For this review, use the dimensioned drawing (mm, ordinates from the lowest corner) and the shaded views. A direction names the side the tool comes from. Round coordinates to 2 decimals unless told otherwise and drop trailing zeros. Write each loop counter-clockwise with the first axis right and the second up, starting at its lowest first coordinate (ties: lowest second). Pieces come first, ordered by that corner, then holes. Notation, with made-up numbers: M 41,-27 L 84,-27 A29 cw 84,-4 Z; hole C 17,34.5 d5. An arc over 180 degrees is marked long. Use one line per item in the form item = value. Start each with the question number.
Item 1: Add section C-C (x = 63.5). State the section outline as (y, z) points (3 decimals), and give its area (3 significant figures).
Item 2: Add section B-B (x = 47). State the section outline as (y, z) points.
Item 3: For line 1 (Z direction, x = 63.5, y = 1.75) (3 decimals); line 2 (Z direction, x = 63.5, y = 22.5); line 3 (Y direction, x = 27, z = 11.5), list the stretches that pass through material, from the lowest coordinate up. Write a range as [from, to].
Item 4: Add section A-A (z = 60.96). State the section outline as (x, y) points (3 decimals).
Item 5: For P1, Ø8, axis at x = 61, z = 35.5, coming from the +Y side; P2, Ø7, axis at y = 3.5, z = 52.5, coming from the -X side; P3, Ø4, axis at x = 31.5, y = 20, coming from the +Z side, all flat-tipped, find the tip position at first contact; note any pin that passes through.
Item 6: Add section D-D (z = 8). State the section outline as (x, y) points.
Item 7: Draft analysis for pull direction Z (two halves, no side actions). For the marked faces 1, 2 and 3, state which applies: released by +Z, released by -Z, zero draft, split by the parting line, or undercut.
Item 8: For the marked faces 4, 5, 6 and 7, list the 3-axis set-ups (+Z, -Z, +X, -X, +Y, -Y) from which the entire face can be reached by the end or side of a thin tool; tool diameter is ignored.
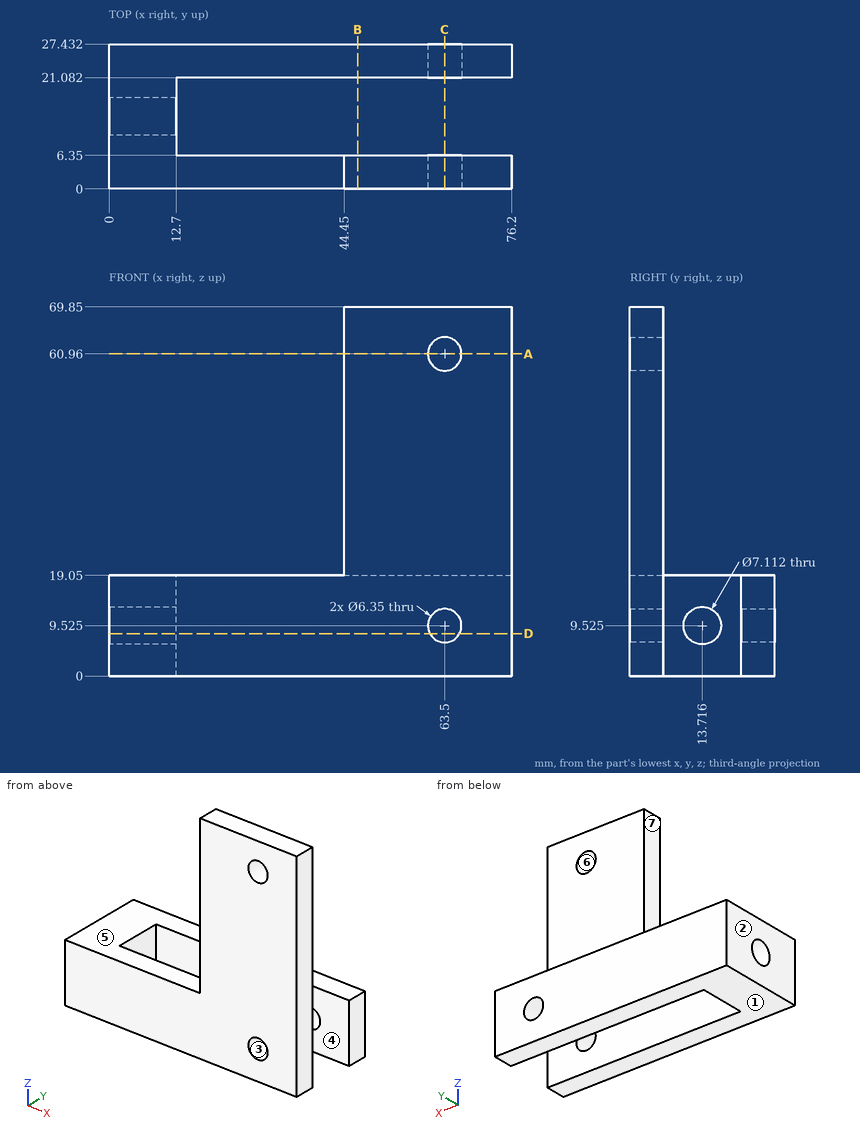
Calculated:
q1.outline = M 0,0 L 6.35,0 L 6.35,6.35 L 0,6.35 Z; M 0,12.7 L 6.35,12.7 L 6.35,57.785 L 0,57.785 Z; M 0,64.135 L 6.35,64.135 L 6.35,69.85 L 0,69.85 Z; M 21.082,0 L 27.432,0 L 27.432,6.35 L 21.082,6.35 Z; M 21.082,12.7 L 27.432,12.7 L 27.432,19.05 L 21.082,19.05 Z
q1.area = 444 mm^2
q2.outline = M 0,0 L 6.35,0 L 6.35,69.85 L 0,69.85 Z; M 21.08,0 L 27.43,0 L 27.43,19.05 L 21.08,19.05 Z
q3.line_1 = [0, 6.35], [12.7, 57.785], [64.135, 69.85]
q3.line_2 = [0, 6.35], [12.7, 19.05]
q3.line_3 = [0, 6.35], [21.08, 27.43]
q4.outline = M 44.45,0 L 60.325,0 L 60.325,6.35 L 44.45,6.35 Z; M 66.675,0 L 76.2,0 L 76.2,6.35 L 66.675,6.35 Z
q5.P1 = 6.35
q5.P2 = 44.45
q5.P3 = 19.05
q6.outline = M 0,0 L 60.72,0 L 60.72,6.35 L 12.7,6.35 L 12.7,10.5 L 0,10.5 Z; M 0,16.93 L 12.7,16.93 L 12.7,21.08 L 60.72,21.08 L 60.72,27.43 L 0,27.43 Z; M 66.28,0 L 76.2,0 L 76.2,6.35 L 66.28,6.35 Z; M 66.28,21.08 L 76.2,21.08 L 76.2,27.43 L 66.28,27.43 Z
q7.face_1 = released by -Z
q7.face_2 = zero draft
q7.face_3 = undercut
q8.face_4 = +Z, -Z, +X
q8.face_5 = +Z, -X, +Y
q8.face_6 = +Y, -Y
q8.face_7 = +Z, -X, +Y, -Y
